Geometry: final body of the model. Coordinates: model frame, mm. A direction names the side the tool comes from. Round coordinates to 2 decimals unless told otherwise and drop trailing zeros. Write each loop counter-clockwise with the first axis right and the second up, starting at its lowest first coordinate (ties: lowest second). Pieces come first, ordered by that corner, then holes. Notation, with made-up numbers: (34.5, 3.25) - (92.5, 3.25) arc R15 ccw to (92.5, 23.25) - close; hole circle Ø11 at (4.25, -29.75). An arc over 180 degrees is marked (long way). Write each question's results on one line, items separated by ' | '.
from build123d import *

# Parameters (mm, degrees)
AUFSATZ_LINEAR_AUSTRAGEN1_DEPTH                      = 10
SKIZZE4_W                                            = 4.9
SKIZZE4_H                                            = 20
AUFSATZ_LINEAR_AUSTRAGEN2_DEPTH                      = 2
STIRNSENKUNG_F_R_M4_ZYLINDERSCHRAUBE_MIT_D           = 4.5
STIRNSENKUNG_F_R_M4_ZYLINDERSCHRAUBE_MIT_CBORE_D     = 8
STIRNSENKUNG_F_R_M4_ZYLINDERSCHRAUBE_MIT_CBORE_DEPTH = 16
F_4_0_4_DURCHMESSER_BOHRUNG1_D                       = 4
FASE1_SIZE                                           = 1


with BuildPart() as part:
    # Skizze1 → Aufsatz-Linear austragen1 (new body, symmetric)
    with BuildSketch(Plane(origin=(0, 0, 0), x_dir=(1, 0, 0), z_dir=(0, 1, 0))):
        with BuildLine():
            ThreePointArc((-10.534455372, 15.89114714), (-16.430025091, 9.672516887), (-19.006664816, 1.5))
            Line((-19.006664816, 1.5), (-12.006664816, 1.5))
            ThreePointArc((-12.006664816, 1.5), (0, 12.1), (12.006664816, 1.5))
            Line((12.006664816, 1.5), (19.006664816, 1.5))
            ThreePointArc((19.006664816, 1.5), (16.430025091, 9.672516887), (10.534455372, 15.89114714))
            Line((10.534455372, 15.89114714), (10, 22))
            Line((10, 22), (-10, 22))
            Line((-10, 22), (-10.534455372, 15.89114714))
        make_face()
    extrude(amount=AUFSATZ_LINEAR_AUSTRAGEN1_DEPTH, both=True)

    # Skizze4 → Aufsatz-Linear austragen2 (add)
    with BuildSketch(Plane(origin=(0, 0, -22), x_dir=(-1, 0, 0), z_dir=(0, 0, -1))):
        Rectangle(SKIZZE4_W, SKIZZE4_H)
    extrude(amount=AUFSATZ_LINEAR_AUSTRAGEN2_DEPTH)

    # Stirnsenkung für M4 Zylinderschraube mit Innensechskant1 (through all)
    with Locations(Plane.XY.offset(-1.5)):
        with Locations((0, 0)):
            CounterBoreHole(STIRNSENKUNG_F_R_M4_ZYLINDERSCHRAUBE_MIT_D / 2, STIRNSENKUNG_F_R_M4_ZYLINDERSCHRAUBE_MIT_CBORE_D / 2, STIRNSENKUNG_F_R_M4_ZYLINDERSCHRAUBE_MIT_CBORE_DEPTH)

    # Ø4.0 (4) Durchmesser Bohrung1 (through all)
    with Locations(Plane.XY.offset(-1.5)):
        with Locations((-15.506664816, 0), (15.506664816, 0)):
            Hole(F_4_0_4_DURCHMESSER_BOHRUNG1_D / 2)

    # Fase1
    fase1_edges = [part.edges().sort_by_distance(p)[0] for p in [
        (0, -10, -12.1),
        (-16.430025091, -10, -9.672516887),
        (16.430025091, -10, -9.672516887),
        (-16.430025091, 10, -9.672516887),
        (0, 10, -12.1),
        (16.430025091, 10, -9.672516887),
    ]]
    chamfer(fase1_edges, length=FASE1_SIZE)


solid = part.part
Q1. Mould query, pull axis Y, two halves, no side actions, for faces 4 (the flat face through (-2.45, 0, -23)), 5 (the cylindrical face through (-13.51, 0.09, -6.23)), 6 (the conical face through (15.776, -9.826, -9.153)). Classes: pulls with the +Y half, pulls with the -Y half, needs draft (parallel to the pull), parting line crosses it, or undercut.
Answer block:
face 4: needs draft | face 5: undercut | face 6: pulls with the -Y half
Q2. Section query D-D, the plane z = -21. Return loops of the section in (x, y), plus the area to 3 significant figures.
Answer block:
outline: (-10.09, -10) - (10.09, -10) - (10.09, 10) - (-10.09, 10) - close; hole circle Ø4.5 at (0, 0) | area: 388 mm2
Q3. Section query C-C, the plane y = 0.75. Return loops of the section in (x, z), plus the area to 3 significant figures.
Answer block:
outline: (-19.01, -1.5) arc R19.07 ccw to (-17.36, -7.88) - (-17.36, -1.5) - close; (-13.65, -13.31) arc R19.07 ccw to (-10.53, -15.89) - (-10, -22) - (-2.45, -22) - (-2.45, -24) - (-2.12, -24) - (-2.12, -17.5) - (-3.93, -17.5) - (-3.93, -11.44) arc R12.1 cw to (-12.01, -1.5) - (-13.65, -1.5) - close; (2.12, -24) - (2.45, -24) - (2.45, -22) - (10, -22) - (10.53, -15.89) arc R19.07 ccw to (13.65, -13.31) - (13.65, -1.5) - (12.01, -1.5) arc R12.1 cw to (3.93, -11.44) - (3.93, -17.5) - (2.12, -17.5) - close; (17.36, -7.88) arc R19.07 ccw to (19.01, -1.5) - (17.36, -1.5) - close | area: 268 mm2
Q4. Access query for faces 1 (the flat face through (0.6, 2.4, -24)), 2 (the flat face through (2, -2, -17.5)), 3 (the flat face through (6, 0, -22)). Directions: +Z, -Z, +X, -X, +Y, -Y. A direction counts if a zero-diameter tool reaches every point of the face in a straight line with its end or side. Return the directions, or none.
Answer block:
face 1: -Z, +X, -X, +Y, -Y | face 2: +Z | face 3: -Z, +X, +Y, -Y
Q5. Section query A-A, the plane x = 0. Return loops of the section in (y, z).
Answer block:
outline: (-10, -24) - (-2.25, -24) - (-2.25, -17.5) - (-4, -17.5) - (-4, -12.1) - (-9, -12.1) - (-10, -13.1) - close; (2.25, -24) - (10, -24) - (10, -13.1) - (9, -12.1) - (4, -12.1) - (4, -17.5) - (2.25, -17.5) - close
Q6. Section query B-B, the plane y = 8.25. Return loops of the section in (x, z), plus the area to 3 significant figures.
Answer block:
outline: (-19.01, -1.5) arc R19.07 ccw to (-10.53, -15.89) - (-10, -22) - (-2.45, -22) - (-2.45, -24) - (2.45, -24) - (2.45, -22) - (10, -22) - (10.53, -15.89) arc R19.07 ccw to (19.01, -1.5) - (12.01, -1.5) arc R12.1 cw to (-12.01, -1.5) - close | area: 410 mm2
Q7. Pin query (flat end, axial travel): pin 1 (9 mm diameter, centred on x = 0.5, y = -1.5, fed in from +Z); pin 2 (1.6 mm diameter, centred on y = 1.5, z = -23.5, fed in from +X); pin 3 (1.5 mm diameter, centred on x = 8, y = -1, fed in from +Z). Return the tip coordinate at first contact, or that it passes through.
Answer block:
pin 1: z = -11.02 | pin 2: x = 2.45 | pin 3: z = -8.36
Q8. Ray query, line 1 along Y through (x, z) = (0, -22.5); line 2 along X through (y, z) = (0, -6.25); line 3 along X through (y, z) = (0, -5.75). Return the intervals inside material, ascending.
Answer block:
line 1: -10 to -2.25, 2.25 to 10 | line 2: -18.01 to -17.51, -13.51 to -10.36, 10.36 to 13.51, 17.51 to 18.01 | line 3: -18.18 to -17.51, -13.51 to -10.65, 10.65 to 13.51, 17.51 to 18.18
